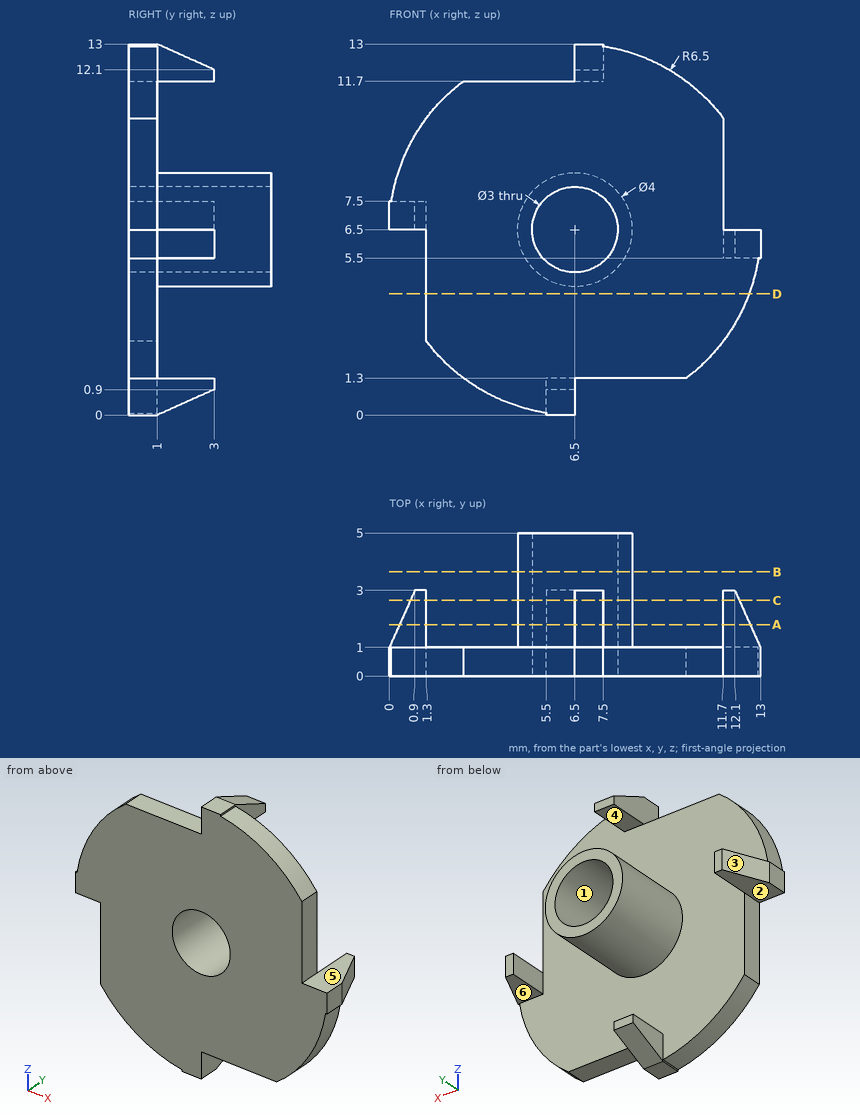
Source: three-view drawing plus pictorial views. Frame: mm from the lowest corner of the part. A direction names the side the tool comes from. Coordinates: 2 decimals unless noted, no trailing zeros. Write each loop counter-clockwise with the first axis right and the second up, starting at its lowest first coordinate (ties: lowest second). Pieces come first, ordered by that corner, then holes. Notation, with made-up numbers: (83.5, 38) -> (127.5, 38) arc R12 ccw to (127.5, 44) -> close; hole circle Ø8 at (20, -21). An arc over 180 degrees is marked (long way). Write each question's results on one line, items separated by ' | '.
Item 1: Mould query, pull axis X, two halves, no side actions, for the marked faces 1, 2 and 3. Classes: +X half, -X half, draft (parallel to the pull), parting line (faces both ways), or undercut.
Conclusion:
face 1: undercut | face 2: draft | face 3: -X half
Item 2: Section query A-A on y = 1.8. Return loops of the section in (x, z), plus the area to 3 significant figures.
Conclusion:
outline: (0.36, 6.5) -> (1.3, 6.5) -> (1.3, 7.5) -> (0.36, 7.5) -> close; circle Ø4 at (6.5, 6.5); (5.5, 0.36) -> (6.5, 0.36) -> (6.5, 1.3) -> (5.5, 1.3) -> close; (6.5, 11.7) -> (7.5, 11.7) -> (7.5, 12.64) -> (6.5, 12.64) -> close; (11.7, 5.5) -> (12.64, 5.5) -> (12.64, 6.5) -> (11.7, 6.5) -> close; hole circle Ø3 at (6.5, 6.5) | area: 9.26 mm^2
Item 3: Section query C-C on y = 2.65. Return loops of the section in (x, z), plus the area to 3 significant figures.
Conclusion:
outline: (0.74, 6.5) -> (1.3, 6.5) -> (1.3, 7.5) -> (0.74, 7.5) -> close; circle Ø4 at (6.5, 6.5); (5.5, 0.74) -> (6.5, 0.74) -> (6.5, 1.3) -> (5.5, 1.3) -> close; (6.5, 11.7) -> (7.5, 11.7) -> (7.5, 12.26) -> (6.5, 12.26) -> close; (11.7, 5.5) -> (12.26, 5.5) -> (12.26, 6.5) -> (11.7, 6.5) -> close; hole circle Ø3 at (6.5, 6.5) | area: 7.73 mm^2
Item 4: Material intervals for probe 1 along Y at (x, z) = (4.5, 7.5); probe 2 along Z at (x, y) = (6.25, 2.5) (3 decimals); probe 3 along X at (y, z) = (3.1, 6.5), sorted ascending.
Conclusion:
probe 1: y = 0 to 1 | probe 2: z = 0.675 to 1.3, 4.516 to 5.021, 7.979 to 8.484 | probe 3: x = 4.5 to 5, 8 to 8.5
Item 5: Set-up query: the marked faces 4, 5 and 6. Return all of +Z, -Z, +X, -X, +Y, -Y with unobstructed straight access to the full face (end or side cutting, diameter ignored); none if empty.
Conclusion:
face 4: +X, -X, +Y | face 5: +Z, +X, +Y, -Y | face 6: -Z, +X, +Y
Item 6: Section query D-D on z = 4.25. Return loops of the section in (x, y).
Conclusion:
outline: (1.3, 0) -> (12.6, 0) -> (12.6, 1) -> (1.3, 1) -> close
Item 7: Pin query (flat end, axial travel): pin 1 Ø0.5 at (y, z) = (1.5, 6) entering from -X; pin 2 Ø0.6 at (x, y) = (0.5, 1.5) entering from +Z; pin 3 Ø3 at (y, z) = (1.5, 3.5) entering from +X; pin 4 Ø1 at (x, z) = (5.5, 3.5) entering from -Y. Return the tip coordinate at first contact, or that it passes through.
Conclusion:
pin 1: stops at x = 4.52 | pin 2: stops at z = 7.5 | pin 3: stops at x = 12.8 | pin 4: stops at y = 0
Item 8: Section query B-B on y = 3.65. Return loops of the section in (x, z).
Conclusion:
outline: circle Ø4 at (6.5, 6.5); hole circle Ø3 at (6.5, 6.5)
